```python
from build123d import *

# Parameters (mm, degrees)
SKETCH1_W                        = 863.6
SKETCH1_H                        = 704.85
BOSS_EXTRUDE1_DEPTH              = 3.175
SKETCH2_W                        = 711.2
SKETCH2_H                        = 603.25
CUT_EXTRUDE1_DEPTH               = 1115.732507432
LPATTERN4_COUNT                  = 6
LPATTERN4_PITCH                  = 127
LPATTERN4_COUNT_DIR2             = 2
LPATTERN4_PITCH_DIR2             = 666.75
LPATTERN5_COUNT                  = 5
LPATTERN5_PITCH                  = 127
F_21_64_0_32813_DIAMETER_HOLE1_D = 8.334502
LPATTERN6_COUNT                  = 2
LPATTERN6_PITCH                  = 736.6
LPATTERN6_COUNT_DIR2             = 2
LPATTERN6_PITCH_DIR2             = 628.65
F_21_64_0_32813_DIAMETER_HOLE2_D = 8.334502
LPATTERN7_COUNT                  = 5
LPATTERN7_PITCH                  = 127
LPATTERN7_COUNT_DIR2             = 2
LPATTERN7_PITCH_DIR2             = 628.65
F_21_64_0_32813_DIAMETER_HOLE3_D = 8.334502
LPATTERN8_COUNT                  = 4
LPATTERN8_PITCH                  = 127
LPATTERN8_COUNT_DIR2             = 2
LPATTERN8_PITCH_DIR2             = 736.6
FILLET1_R                        = 6.35
LPATTERN9_COUNT                  = 5
LPATTERN9_PITCH                  = 127


with BuildPart() as part:
    # Sketch1 → Boss-Extrude1 (new body)
    with BuildSketch(Plane.XY):
        with Locations((431.8, 352.425)):
            Rectangle(SKETCH1_W, SKETCH1_H)
    extrude(amount=BOSS_EXTRUDE1_DEPTH)

    # Sketch2 → Cut-Extrude1 (cut, through all)
    with BuildSketch(Plane.XY.offset(3.175)):
        with Locations((406.4, 352.425)):
            Rectangle(SKETCH2_W, SKETCH2_H)
    extrude(amount=-CUT_EXTRUDE1_DEPTH, mode=Mode.SUBTRACT)

    # Sketch12 → CSK for 1/4 Flat Head Machine Screw2 (revolve, cut)
    with BuildSketch(Plane(origin=(114.3, 19.05, 0), x_dir=(0, 1, 0), z_dir=(1, 0, 0))):
        Polygon((0, 0), (0, 3.175), (3.3782, 3.175), (3.3782, 3.520932584), (6.4389, 0), align=None)
    csk_for_1_4_flat_head_machine_screw2 = revolve(axis=Axis((114.3, 19.05, -6.35), (0, 0, 1)), mode=Mode.SUBTRACT)

    # LPattern4: CSK for 1_4 Flat Head Machine Screw2 6 × 2
    with Locations(*[(i * LPATTERN4_PITCH, j * LPATTERN4_PITCH_DIR2, 0) for i in range(LPATTERN4_COUNT) for j in range(LPATTERN4_COUNT_DIR2) if (i, j) != (0, 0)]):
        add(csk_for_1_4_flat_head_machine_screw2, mode=Mode.SUBTRACT)

    # Sketch14 → CSK for 1/4 Flat Head Machine Screw3 (revolve, cut)
    with BuildSketch(Plane(origin=(25.4, 98.425, 0), x_dir=(0, 1, 0), z_dir=(1, 0, 0))):
        Polygon((0, 0), (0, 3.175), (3.3782, 3.175), (3.3782, 3.520932584), (6.4389, 0), align=None)
    csk_for_1_4_flat_head_machine_screw3 = revolve(axis=Axis((25.4, 98.425, -6.35), (0, 0, 1)), mode=Mode.SUBTRACT)

    # LPattern5: CSK for 1/4 Flat Head Machine Screw3 ×5
    with Locations(*[(0, i * LPATTERN5_PITCH, 0) for i in range(1, LPATTERN5_COUNT)]):
        add(csk_for_1_4_flat_head_machine_screw3, mode=Mode.SUBTRACT)

    # 21/64 (0.32813) Diameter Hole1 (through all)
    with Locations(Plane(origin=(0, 0, 0), x_dir=(-1, 0, 0), z_dir=(0, 0, -1))):
        with Locations((-38.1, 38.1)):
            f_21_64_0_32813_diameter_hole1 = Hole(F_21_64_0_32813_DIAMETER_HOLE1_D / 2)

    # LPattern6: 21_64 _0.32813_ Diameter Hole1 2 × 2
    with Locations(*[(i * LPATTERN6_PITCH, j * LPATTERN6_PITCH_DIR2, 0) for i in range(LPATTERN6_COUNT) for j in range(LPATTERN6_COUNT_DIR2) if (i, j) != (0, 0)]):
        add(f_21_64_0_32813_diameter_hole1, mode=Mode.SUBTRACT)

    # 21/64 (0.32813) Diameter Hole2 (through all)
    with Locations(Plane(origin=(0, 0, 0), x_dir=(-1, 0, 0), z_dir=(0, 0, -1))):
        with Locations((-177.8, 38.1)):
            f_21_64_0_32813_diameter_hole2 = Hole(F_21_64_0_32813_DIAMETER_HOLE2_D / 2)

    # LPattern7: 21_64 _0.32813_ Diameter Hole2 5 × 2
    with Locations(*[(i * LPATTERN7_PITCH, j * LPATTERN7_PITCH_DIR2, 0) for i in range(LPATTERN7_COUNT) for j in range(LPATTERN7_COUNT_DIR2) if (i, j) != (0, 0)]):
        add(f_21_64_0_32813_diameter_hole2, mode=Mode.SUBTRACT)

    # 21/64 (0.32813) Diameter Hole3 (through all)
    with Locations(Plane(origin=(0, 0, 0), x_dir=(-1, 0, 0), z_dir=(0, 0, -1))):
        with Locations((-38.1, 161.925)):
            f_21_64_0_32813_diameter_hole3 = Hole(F_21_64_0_32813_DIAMETER_HOLE3_D / 2)

    # LPattern8: 21_64 _0.32813_ Diameter Hole3 4 × 2
    with Locations(*[(j * LPATTERN8_PITCH_DIR2, i * LPATTERN8_PITCH, 0) for i in range(LPATTERN8_COUNT) for j in range(LPATTERN8_COUNT_DIR2) if (i, j) != (0, 0)]):
        add(f_21_64_0_32813_diameter_hole3, mode=Mode.SUBTRACT)

    # Fillet1
    fillet1_edges = [part.edges().sort_by_distance(p)[0] for p in [
        (50.8, 50.8, 1.5875),
        (50.8, 654.05, 1.5875),
        (762, 654.05, 1.5875),
        (762, 50.8, 1.5875),
    ]]
    fillet(fillet1_edges, radius=FILLET1_R)

    # Sketch22 → CSK for #8 Flat Head Machine Screw1 (revolve, cut)
    with BuildSketch(Plane(origin=(774.7, 606.425, 0), x_dir=(0, 1, 0), z_dir=(1, 0, 0))):
        Polygon((0, 0), (0, 3.175), (2.2479, 3.175), (2.2479, 2.26450021), (4.2164, 0), align=None)
    csk_for_8_flat_head_machine_screw1 = revolve(axis=Axis((774.7, 606.425, -6.35), (0, 0, 1)), mode=Mode.SUBTRACT)

    # LPattern9: CSK for #8 Flat Head Machine Screw1 ×5
    with Locations(*[(0, -i * LPATTERN9_PITCH, 0) for i in range(1, LPATTERN9_COUNT)]):
        add(csk_for_8_flat_head_machine_screw1, mode=Mode.SUBTRACT)


solid = part.part
```
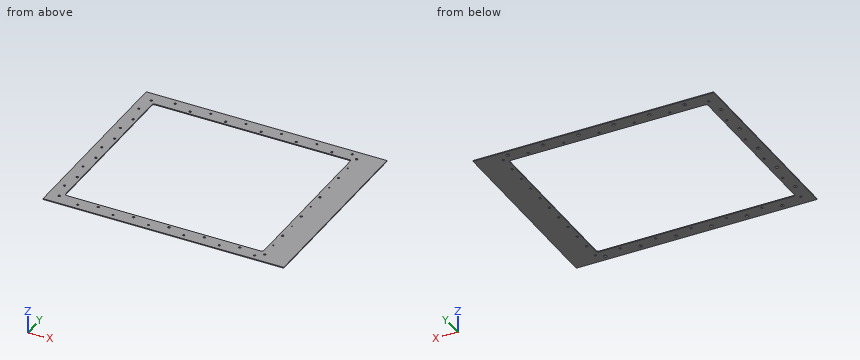
Read the model definition and answer for the solid it produces. Units are mm, in the model's axes. Give positions to 0.01 mm unless a question says otherwise; leave off trailing zeros. Write each loop counter-clockwise with the first axis right and the second up, starting at its lowest first coordinate (ties: lowest second). Pieces come first, ordered by that corner, then holes. Notation, with made-up numbers: (14.5, 0) - (27.5, 0) arc R20 ccw to (27.5, 29) - close; hole circle Ø1 at (74, 41). An arc over 180 degrees is marked (long way). Write item = value, one per line. Start each with the question number.
Item 1: This flat-tipped pin is pushed along its axis until it touches: P1, Ø13.5, axis at x = 38.1, y = 542.925, coming from the +Z side (3 decimals). Where does it stop, or does it pass through?
Item 2: Find the intervals of material crossed by probe 1 along X at (y, z) = (382, 1.7); probe 2 along Y at (x, z) = (629, 0.25); probe 3 along X at (y, z) = (350.5, 1.65), in increasing order. Write a range as [from, to].
Item 3: Find section A-A (x = 661.5). Give the vertices of the cut face in (y, z) (3 decimals), then the cut area to 3 significant figures.
Item 4: Find section C-C (z = 1.6). State how many separate pieces and enclosed holes the cut face has, then the cut area to 3 significant figures.
Item 5: Find section B-B (y = 402). Give the vertices of the cut face in (x, z) (3 decimals).
Response:
q1.P1 = 3.175
q2.probe_1 = [0, 50.8], [762, 863.6]
q2.probe_2 = [0, 50.8], [654.05, 704.85]
q2.probe_3 = [0, 20.78], [30.02, 50.8], [762, 772.69], [776.71, 863.6]
q3.outline = (0, 0) - (50.8, 0) - (50.8, 3.175) - (0, 3.175) - close; (654.05, 0) - (704.85, 0) - (704.85, 3.175) - (654.05, 3.175) - close
q3.area = 323 mm²
q4.separate_pieces = 1
q4.enclosed_holes = 45
q4.area = 177,000 mm²
q5.outline = (0, 0) - (50.8, 0) - (50.8, 3.175) - (0, 3.175) - close; (762, 0) - (863.6, 0) - (863.6, 3.175) - (762, 3.175) - close
